from build123d import *

# Parameters (mm, degrees)
F2_SIZE = 5.08
F3_SIZE = 2.54


with BuildPart() as f1:
    # F0 (on Front) → F1 (revolve)
    with BuildSketch(Plane.XZ):
        with BuildLine():
            Line((0, 88.4301), (0, 109.5375))
            Line((0, 109.5375), (-152.4, 109.5375))
            Line((-152.4, 109.5375), (-152.4, 47.625))
            Line((-152.4, 47.625), (-114.3, 47.625))
            Line((-114.3, 47.625), (-114.3, 75.7301))
            ThreePointArc((-114.3, 75.7301), (-110.580256, 84.710356), (-101.6, 88.4301))
            Line((-101.6, 88.4301), (0, 88.4301))
        make_face()
    revolve(axis=Axis((-61.485236, 0, 0), (-1, 0, 0)))

    # F2
    f2_edges = [f1.edges().sort_by_distance(p)[0] for p in [
        (-152.4, 0, -109.5375),
    ]]
    chamfer(f2_edges, length=F2_SIZE)

    # F3
    f3_edges = [f1.edges().sort_by_distance(p)[0] for p in [
        (-152.4, 0, -47.625),
        (-114.3, 0, -47.625),
        (-133.35, 0, 47.625),
    ]]
    chamfer(f3_edges, length=F3_SIZE)


solid = f1.part
Design review of the part built by this model. Coordinates are the model's own, in mm. A direction names the side the tool comes from. Coordinates: 2 decimals unless noted, no trailing zeros. Order: outer loops, then holes, each group sorted by start corner. A loop starts at its lowest first (then second) coordinate and runs counter-clockwise, first axis right, second up. Notation, with made-up numbers: (-16, 30.25) -> (23, 30.25) arc R29 ccw to (23, 55.25) -> close; hole circle Ø5 at (3, 34). An arc over 180 degrees is marked (long way). One line per item, written item: value.
1) Draft analysis for pull direction Y (two halves, no side actions). For faces 1 (the face through (0, 49, 74)), 2 (the face through (-50.089, -86.327, -19.17)), 3 (the face through (-74.7, 108.6, -14.3)), state which applies: +Y half, -Y half, draft (parallel to the pull), parting line (faces both ways), or undercut.
Output values:
face 1: draft
face 2: undercut
face 3: parting line
2) To check wall thickness, follow probe 1 along Y at (x, z) = (-61, 0); probe 2 along Y at (x, z) = (-131, 0) (1 decimal); probe 3 along X at (y, z) = (-21.5, -49.5). State the ranges of each line that lie inside material, in increasing order. Write a range as [from, to].
Output values:
probe 1: y = [-109.54, -88.43], [88.43, 109.54]
probe 2: y = [-109.5, -47.6], [47.6, 109.5]
probe 3: x = [-152.4, -114.3]
3) Machinability: for faces 4 (the face through (-114.3, -16, -49)), 5 (the face through (-152.153, -102.214, -22.698)), which of the approach directions +Z, -Z, +X, -X, +Y, -Y give a long, thin tool a straight path to every point of the face, cutting with its end or side? Answer none if there is none.
Output values:
face 4: +X
face 5: -X
4) Clearance check with flat-ended pins moving along their axes: P1, Ø12, axis at y = -84.5, z = 82.5, coming from the +X side; P2, Ø6, axis at x = -40.5, y = 18, coming from the -Z side; P3, Ø8, axis at x = -90, y = -25, coming from the +Z side; P4, Ø4, axis at x = -79, y = 17, coming from the +Z side. State where each tip first meets the part, or that it passes through.
Output values:
P1: passes through
P2: stops at z = -108.51
P3: stops at z = 107.51
P4: stops at z = 108.51
5) We need section C-C, the plane x = -14. Give the boundary of the cut face in (y, z) (1 decimal), then the cut area to 3 significant figures.
Output values:
outline: circle Ø219.1 at (0, 0); hole circle Ø176.9 at (0, 0)
area: 13,100 mm2
6) We need section A-A, the plane z = 0. Give the boundary of the cut face in (x, y) (1 decimal), then the cut area to 3 significant figures.
Output values:
outline: (-152.4, -104.5) -> (-147.3, -109.5) -> (0, -109.5) -> (0, -88.4) -> (-101.6, -88.4) arc R12.7 cw to (-114.3, -75.7) -> (-114.3, -50.2) -> (-116.8, -47.6) -> (-149.9, -47.6) -> (-152.4, -50.2) -> close; (-152.4, 50.2) -> (-149.9, 47.6) -> (-116.8, 47.6) -> (-114.3, 50.2) -> (-114.3, 75.7) arc R12.7 cw to (-101.6, 88.4) -> (0, 88.4) -> (0, 109.5) -> (-147.3, 109.5) -> (-152.4, 104.5) -> close
area: 9,570 mm2
